Check sheet for the modelled part. Datum: model origin and axes. Units: mm. A direction names the side the tool comes from. Round coordinates to 2 decimals unless told otherwise and drop trailing zeros. Write each loop counter-clockwise with the first axis right and the second up, starting at its lowest first coordinate (ties: lowest second). Pieces come first, ordered by that corner, then holes. Notation, with made-up numbers: (31.25, 48.25) - (39.25, 48.25) arc R14 cw to (39.25, 53.25) - close; hole circle Ø9 at (25, 21.5). An arc over 180 degrees is marked (long way). Answer as a JSON object with one key per item and string values. Group by question number.
Item 1: Gauge pin test, flat ends, axial feed: P1, Ø1, axis at x = -2, y = 0, coming from the +Z side; P2, Ø1.6, axis at y = 2, z = 7, coming from the -X side (3 decimals); P3, Ø0.7, axis at y = 2, z = 7, coming from the +X side (3 decimals); P4, Ø1.1, axis at x = -9.51, z = 4.09, coming from the -Y side. Record the tip position at first contact, or that the pin passes through.
Item 2: Release check for a two-part mould opening along X. For faces 1 (the flat face through (0, -1, 1)), 2 (the flat face through (4, -0.5, 4)), 3 (the cylindrical face through (5.981, 0.394, -10.403)), 4 (the cylindrical face through (-5.37, 0.39, 10.73)) record: pulls with the +X half, pulls with the -X half, needs draft (parallel to the pull), parting line crosses it, or undercut.
Item 3: Sectioned sample at D-D on x = -4.5. Record the boundary of the cut face in (y, z).
Item 4: Sectioned sample at A-A on x = -7.5. Record the boundary of the cut face in (y, z).
Item 5: Set-up check for faces 5 (the flat face through (5.725, 2, 7)), 6 (the flat face through (-4, -0.5, 4)), 7 (the flat face through (8.28, -1, 4)), 8 (the flat face through (0.1, -0.5, 2)): record each of +Z, -Z, +X, -X, +Y, -Y from which the full face is reachable in a straight line by a thin tool's end or side.
Item 6: Thickness scan on line 1 (Y direction, x = -3, z = 6.25); line 2 (Y direction, x = -0.25, z = 4); line 3 (Y direction, x = -5.5, z = -4.25). Record the ranges inside material, lowest first.
Item 7: Sectioned sample at B-B on x = 0. Record the boundary of the cut face in (y, z).
Item 8: Sectioned sample at C-C on z = -8.5. Record the boundary of the cut face in (x, y), plus the area to 3 significant figures.
```python
from build123d import *

# Parameters (mm, degrees)
SKETCH1_R           = 12
BOSS_EXTRUDE1_DEPTH = 0.8
CUT_EXTRUDE1_START  = -0.8
CUT_EXTRUDE1_DEPTH  = 0.8
SKETCH3_R           = 0.6
SKETCH3_R_2         = 0.3
CUT_EXTRUDE2_DEPTH  = 0.8
SKETCH4_W           = 8
SKETCH4_H           = 4
BOSS_EXTRUDE2_DEPTH = 1
SKETCH5_R           = 8
BOSS_EXTRUDE3_DEPTH = 3.2
SKETCH6_W           = 1.35
SKETCH6_H           = 4
BOSS_EXTRUDE4_DEPTH = 1.8
SKETCH7_W           = 1.25
SKETCH7_H           = 2
BOSS_EXTRUDE5_DEPTH = 1.5
SKETCH8_W           = 1.6
SKETCH8_H           = 2.6
BOSS_EXTRUDE6_DEPTH = 0.55


with BuildPart() as part:
    # Sketch1 → Boss-Extrude1 (new body)
    with BuildSketch(Plane(origin=(0, 0, 0), x_dir=(1, 0, 0), z_dir=(0, 1, 0))):
        with Locations(Location((0, 0, 0), (0, 0, 270))):
            Circle(SKETCH1_R)
    extrude(amount=BOSS_EXTRUDE1_DEPTH)

    # Sketch2 → Cut-Extrude1 (cut)
    with BuildSketch(Plane(origin=(0, 0.8, 0), x_dir=(1, 0, 0), z_dir=(0, 1, 0)).offset(CUT_EXTRUDE1_START)):
        with BuildLine():
            Line((-11.508257905, 3.4), (-9.5, 3.4))
            Line((-9.5, 3.4), (-9.5, 5.4))
            Line((-9.5, 5.4), (-10.71634266, 5.4))
            ThreePointArc((-10.71634266, 5.4), (-11.157204738, 4.417780261), (-11.508257905, 3.4))
        make_face()
        with BuildLine():
            ThreePointArc((0, 12), (-0.500435352, 11.989560645), (-1, 11.958260743))
            Line((-1, 11.958260743), (-1, 10.5))
            Line((-1, 10.5), (1, 10.5))
            Line((1, 10.5), (1, 11.958260743))
            ThreePointArc((1, 11.958260743), (0.500435352, 11.989560645), (0, 12))
        make_face()
        with BuildLine():
            Line((8.6, 5), (10.908712115, 5))
            ThreePointArc((10.908712115, 5), (10.376053526, 6.028060486), (9.746794345, 7))
            Line((9.746794345, 7), (8.6, 7))
            Line((8.6, 7), (8.6, 5))
        make_face()
        with BuildLine():
            Line((9.9, -3.9), (9.9, -6.781592733))
            ThreePointArc((9.9, -6.781592733), (10.721534718, -5.389683969), (11.348568192, -3.9))
            Line((11.348568192, -3.9), (9.9, -3.9))
        make_face()
    extrude(amount=CUT_EXTRUDE1_DEPTH, mode=Mode.SUBTRACT)

    # Sketch3 → Cut-Extrude2 (cut)
    with BuildSketch(Plane(origin=(0, 0.8, 0), x_dir=(1, 0, 0), z_dir=(0, 1, 0))):
        with Locations(Location((-9.505920047, -4.093895952, 0), (0, 0, 270))):
            Circle(SKETCH3_R)
        with Locations(Location((10.702676663, -2.70819354, 0), (0, 0, 270))):
            Circle(SKETCH3_R_2)
        with Locations(Location((10.699796483, -0.804521739, 0), (0, 0, 270))):
            Circle(SKETCH3_R_2)
    extrude(amount=-CUT_EXTRUDE2_DEPTH, mode=Mode.SUBTRACT)

    # Sketch4 → Boss-Extrude2 (add)
    with BuildSketch(Plane(origin=(0, 0, 0), x_dir=(-1, 0, 0), z_dir=(0, -1, 0))):
        with Locations((0, -4)):
            Rectangle(SKETCH4_W, SKETCH4_H)
    extrude(amount=BOSS_EXTRUDE2_DEPTH)

    # Sketch5 → Boss-Extrude3 (add)
    with BuildSketch(Plane(origin=(0, -1, 0), x_dir=(-1, 0, 0), z_dir=(0, -1, 0))):
        with Locations(Location((0, -4, 0), (0, 0, 90))):
            Circle(SKETCH5_R)
    extrude(amount=BOSS_EXTRUDE3_DEPTH)

    # Sketch6 → Boss-Extrude4 (add)
    with BuildSketch(Plane.XZ):
        with Locations((8.955, 4)):
            Rectangle(SKETCH6_W, SKETCH6_H)
    extrude(amount=BOSS_EXTRUDE4_DEPTH)

    # Sketch7 → Boss-Extrude5 (add)
    with BuildSketch(Plane(origin=(0, 0.8, 0), x_dir=(1, 0, 0), z_dir=(0, 1, 0))):
        with Locations((5.1, -6.96)):
            Rectangle(SKETCH7_W, SKETCH7_H)
    extrude(amount=BOSS_EXTRUDE5_DEPTH)

    # Sketch8 → Boss-Extrude6 (add)
    with BuildSketch(Plane(origin=(0, 0.8, 0), x_dir=(1, 0, 0), z_dir=(0, 1, 0))):
        with Locations((7.435, -4.345)):
            Rectangle(SKETCH8_W, SKETCH8_H)
    extrude(amount=BOSS_EXTRUDE6_DEPTH)


solid = part.part
```
Completed:
{
 "1": {"P1": "z = 11.91", "P2": "x = 4.475", "P3": "x = 5.725", "P4": "through"},
 "2": {"face 1": "undercut", "face 2": "undercut", "face 3": "pulls with the +X half", "face 4": "parting line crosses it"},
 "3": {"outline": "(-4.2, -2.61) - (-1, -2.61) - (-1, 10.61) - (-4.2, 10.61) - close; (0, -11.12) - (0.8, -11.12) - (0.8, 11.12) - (0, 11.12) - close"},
 "4": {"outline": "(-4.2, 1.22) - (-1, 1.22) - (-1, 6.78) - (-4.2, 6.78) - close; (0, -9.37) - (0.8, -9.37) - (0.8, 9.37) - (0, 9.37) - close"},
 "5": {"face 5": "+Z, -Z, +X, +Y", "face 6": "+Z, -Z, -X", "face 7": "+Z, -Z, -Y", "face 8": "-Z, +X, -X"},
 "6": {"line 1": "-4.2 to -1, 0 to 0.8", "line 2": "-4.2 to 0.8", "line 3": "0 to 0.8"},
 "7": {"outline": "(-4.2, -4) - (-1, -4) - (-1, 2) - (0, 2) - (0, -10.5) - (0.8, -10.5) - (0.8, 12) - (0, 12) - (0, 6) - (-1, 6) - (-1, 12) - (-4.2, 12) - close"},
 "8": {"outline": "(-8.47, 0) - (8.47, 0) - (8.47, 0.8) - (-8.47, 0.8) - close", "area": "13.6 mm²"}
}
